Study the drawing (mm; zero at the part's minimum x, y, z) and answer. A direction names the side the tool comes from. Round coordinates to 2 decimals unless told otherwise and drop trailing zeros. Order: outer loops, then holes, each group sorted by start corner. A loop starts at its lowest first (then second) coordinate and runs counter-clockwise, first axis right, second up. Notation, with made-up numbers: (8, 58.25) - (32, 58.25) arc R22 cw to (32, 80.25) - close; hole circle Ø7 at (-24, 26). An arc over 180 degrees is marked (long way). Put each result on its own line as item: value.
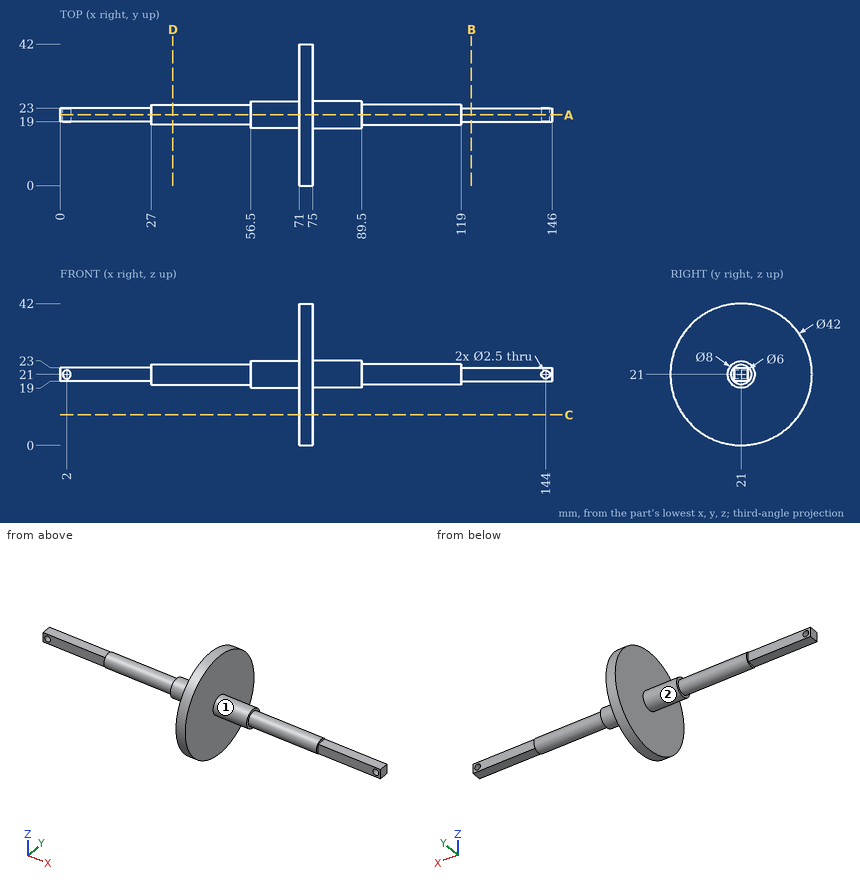
1) A cutting plane is placed at A-A on y = 21. Give the number of separate pieces and of enclosed holes in the cut face, then the cut area to 3 significant figures.
Findings below:
separate pieces: 1
enclosed holes: 2
area: 960 mm2
2) A cutting plane is placed at B-B on x = 122. Write down the section's boundary in (y, z), then the cut area to 3 significant figures.
Findings below:
outline: (19, 19) - (23, 19) - (23, 23) - (19, 23) - close
area: 16.0 mm2
3) Given pin 1 Ø1.2 at (x, z) = (14, 21.5) entering from -Y; pin 2 Ø4.5 at (x, z) = (136.5, 21.5) entering from +Y; pin 3 Ø4.5 at (x, y) = (10.5, 21.5) entering from +Z; pin 4 Ø2 at (x, z) = (144, 21) entering from -Y, each flat-ended and moving along its own axis, determine where each tip first touches the part or whether it passes through.
Findings below:
pin 1: stops at y = 19
pin 2: stops at y = 23
pin 3: stops at z = 23
pin 4: passes through
4) Straight lines are drawn through the part: L1, parallel to X at y = 20.9, z = 21; L2, parallel to Z at x = 144, y = 20.25; L3, parallel to X at y = 10, z = 7. For each, find the intervals that lie inside material, in ascending order. Write a range as from..to.
Findings below:
L1: x = 0..0.75, 3.25..142.75, 145.25..146
L2: z = 19..19.75, 22.25..23
L3: x = 71..75
5) A cutting plane is placed at D-D on x = 33.5. Write down the section's boundary in (y, z), then the cut area to 3 significant figures.
Findings below:
outline: circle Ø6 at (21, 21)
area: 28.3 mm2
6) For the marked faces 1 and 2, determine the directions among +Z, -Z, +X, -X, +Y, -Y from which every point of the face is accessible in a straight line to the end or side of a thin tool.
Findings below:
face 1: +X
face 2: -X
7) A cutting plane is placed at C-C on z = 9. Write down the section's boundary in (x, y), then the cut area to 3 significant figures.
Findings below:
outline: (71, 3.77) - (75, 3.77) - (75, 38.23) - (71, 38.23) - close
area: 138 mm2
